Geometry check sheet. Reference: drawing and pictorial views, mm from the part's lowest x, y, z. Coordinates: 2 decimals unless noted, no trailing zeros. Write each loop counter-clockwise with the first axis right and the second up, starting at its lowest first coordinate (ties: lowest second). Pieces come first, ordered by that corner, then holes. Notation, with made-up numbers: (43.25, 63) -> (90.25, 63) arc R12 cw to (90.25, 72) -> close; hole circle Ø2 at (13, 11.25). An arc over 180 degrees is marked (long way). Use a Markdown table: item, result.
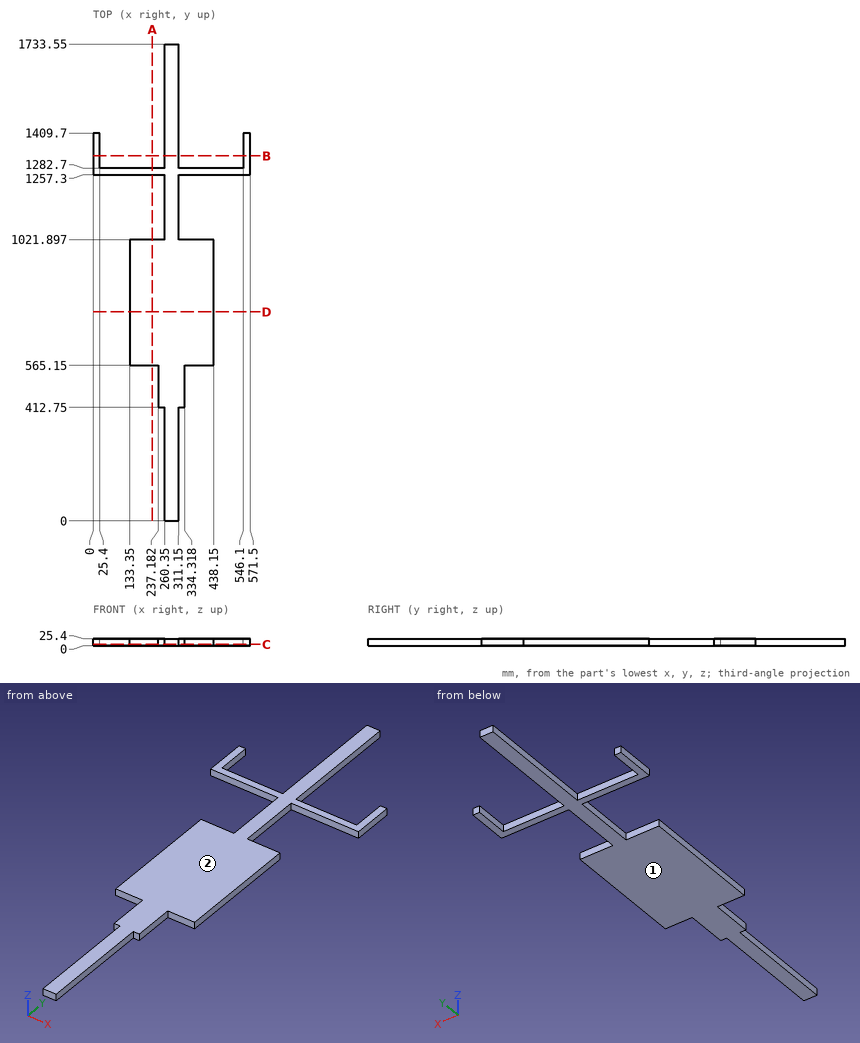
Item 1: Section check A-A on x = 216. Record the boundary of the cut face in (y, z), then the cut area to 3 significant figures.
Answer block:
| item | result |
|---|---|
| outline | (565.15, 0) -> (1021.9, 0) -> (1021.9, 25.4) -> (565.15, 25.4) -> close; (1257.3, 0) -> (1282.7, 0) -> (1282.7, 25.4) -> (1257.3, 25.4) -> close |
| area | 12,200 mm^2 |
Item 2: Thickness scan on L1, parallel to Y at x = 206, z = 24; L2, parallel to X at y = 931.5, z = 14.25; L3, parallel to X at y = 1523, z = 20. Record the ranges inside material, lowest first. Write a range as [from, to].
Answer block:
| item | result |
|---|---|
| L1 | y = [565.15, 1021.9], [1257.3, 1282.7] |
| L2 | x = [133.35, 438.15] |
| L3 | x = [260.35, 311.15] |
Item 3: Section check D-D on y = 760. Record the boundary of the cut face in (x, z).
Answer block:
| item | result |
|---|---|
| outline | (133.35, 0) -> (438.15, 0) -> (438.15, 25.4) -> (133.35, 25.4) -> close |
Item 4: Section check C-C on z = 5. Record the boundary of the cut face in (x, y), then the cut area to 3 significant figures.
Answer block:
| item | result |
|---|---|
| outline | (0, 1257.3) -> (260.35, 1257.3) -> (260.35, 1021.9) -> (133.35, 1021.9) -> (133.35, 565.15) -> (237.18, 565.15) -> (237.18, 412.75) -> (260.35, 412.75) -> (260.35, 0) -> (311.15, 0) -> (311.15, 412.75) -> (334.32, 412.75) -> (334.32, 565.15) -> (438.15, 565.15) -> (438.15, 1021.9) -> (311.15, 1021.9) -> (311.15, 1257.3) -> (571.5, 1257.3) -> (571.5, 1409.7) -> (546.1, 1409.7) -> (546.1, 1282.7) -> (311.15, 1282.7) -> (311.15, 1733.55) -> (260.35, 1733.55) -> (260.35, 1282.7) -> (25.4, 1282.7) -> (25.4, 1409.7) -> (0, 1409.7) -> close |
| area | 231,000 mm^2 |
Item 5: Mould release check, pull along Z, two halves, no side actions. Record for the marked faces 1 and 2: +Z half, -Z half, draft (parallel to the pull), parting line (faces both ways), or undercut.
Answer block:
| item | result |
|---|---|
| face 1 | -Z half |
| face 2 | +Z half |
Item 6: Depth check by flat-ended pin: P1, Ø1, axis at x = 88.5, z = 23, coming from the +Y side; P2, Ø12, axis at x = 81, z = 19.5, coming from the -Y side; P3, Ø12.5, axis at x = 556, z = 16.5, coming from the +Y side. Enter the tip coordinate at first touch or a pass-through.
Answer block:
| item | result |
|---|---|
| P1 | stops at y = 1282.7 |
| P2 | stops at y = 1257.3 |
| P3 | stops at y = 1409.7 |
Item 7: Section check B-B on y = 1327. Record the boundary of the cut face in (x, z), then the cut area to 3 significant figures.
Answer block:
| item | result |
|---|---|
| outline | (0, 0) -> (25.4, 0) -> (25.4, 25.4) -> (0, 25.4) -> close; (260.35, 0) -> (311.15, 0) -> (311.15, 25.4) -> (260.35, 25.4) -> close; (546.1, 0) -> (571.5, 0) -> (571.5, 25.4) -> (546.1, 25.4) -> close |
| area | 2,580 mm^2 |
